from build123d import *

# Parameters (mm, degrees)
SKETCH1_R           = 712.819772368
SKETCH1_R_2         = 636.619772368
TRACKTOP_DEPTH      = 6.35
SKETCH6_R           = 1.8288
MOUNTINGHOLES_DEPTH = 1009.099389076
CIRPATTERN3_COUNT   = 16


with BuildPart() as part:
    # Sketch1 → TrackTop (new body)
    with BuildSketch(Plane(origin=(0, 0, 0), x_dir=(1, 0, 0), z_dir=(0, 1, 0))):
        with Locations(Location((0, 0, 0), (0, 0, 270))):
            Circle(SKETCH1_R)
        with Locations(Location((0, 0, 0), (0, 0, 270))):
            Circle(SKETCH1_R_2, mode=Mode.SUBTRACT)
    extrude(amount=TRACKTOP_DEPTH)

    # Sketch6 → MountingHoles (cut, symmetric)
    with BuildSketch(Plane(origin=(0, 0, 0), x_dir=(1, 0, 0), z_dir=(0, 1, 0))):
        with Locations(Location((649.319772368, 0, 0), (0, 0, 270))):
            Circle(SKETCH6_R)
        with Locations(Location((700.119772368, 0, 0), (0, 0, 270))):
            Circle(SKETCH6_R)
    mountingholes = extrude(amount=MOUNTINGHOLES_DEPTH, both=True, mode=Mode.SUBTRACT)

    # CirPattern3: MountingHoles ×16 about axis
    cirpattern3_axis = Axis((0, 0, 0), (0, 1, 0))
    for i in range(1, CIRPATTERN3_COUNT):
        add(mountingholes.rotate(cirpattern3_axis, i * 360 / CIRPATTERN3_COUNT), mode=Mode.SUBTRACT)


solid = part.part
Can you work these out from the model? Positions are in its coordinate system, mm. Round coordinates to 2 decimals unless told otherwise and drop trailing zeros. Write each loop counter-clockwise with the first axis right and the second up, starting at its lowest first coordinate (ties: lowest second). Pieces come first, ordered by that corner, then holes. Notation, with made-up numbers: (16, 43) - (35, 43) arc R17 ccw to (35, 52) - close; hole circle Ø1 at (6.25, 81.25). An arc over 180 degrees is marked (long way). Write each question's results on one line, items separated by ' | '. Start each with the question number.
1) Suppose I cut it at B-B (y = 1.75). Give the number of separate pieces and of enclosed holes in the cut face, and give its area (3 significant figures).
2) We'd pull the mould along Z, two halves only. Please class faces 1 (the cylindrical face through (-695.87, 3.13, -154.53)), 2 (the flat face through (584, 0, -267)), 3 (the cylindrical face through (-387.37, 3.13, -505.2)): released by +Z, released by -Z, zero draft, split by the parting line, or undercut.
3) Please list where these lines run through material, in increasing order: line 1 (Z direction, x = -438, y = 5.75); line 2 (Z direction, x = 531.5, y = 2.5); line 3 (X direction, y = 1.75, z = -172.5).
4) For pin 1 Ø3.5 at (x, z) = (459.14, 459.14) entering from -Y; pin 2 Ø1 at (y, z) = (4.5, 535.5) entering from -X; pin 3 Ø1 at (y, z) = (2, 90) entering from -X, each with a flat end and sliding along its axis, tell me the tip position at first contact or that it passes through.
5) Suppose I cut it at A-A (x = -355). List the corners of the cut face in (y, z) for me.
6) Suppose I cut it at C-C (x = 128). List the corners of the cut face in (y, z) for me.
Here are the results:
1) separate pieces: 1 | enclosed holes: 33 | area: 323,000 mm2
2) face 1: split by the parting line | face 2: zero draft | face 3: undercut
3) line 1: z = -562.38 to -462, 462 to 562.38 | line 2: z = -474.99 to -350.42, 350.42 to 474.99 | line 3: x = -691.63 to -612.8, 612.8 to 691.63
4) pin 1: passes through | pin 2: stops at x = -471.05 | pin 3: stops at x = -707.18
5) outline: (0, -618.13) - (6.35, -618.13) - (6.35, -528.45) - (0, -528.45) - close; (0, 528.45) - (6.35, 528.45) - (6.35, 618.13) - (0, 618.13) - close
6) outline: (0, -701.23) - (6.35, -701.23) - (6.35, -623.62) - (0, -623.62) - close; (0, 623.62) - (6.35, 623.62) - (6.35, 701.23) - (0, 701.23) - close
